from build123d import *

# Parameters (mm, degrees)
SKETCH1_W           = 12
SKETCH1_H           = 4.5
BOSS_EXTRUDE1_DEPTH = 12.23
BOSS_EXTRUDE2_DEPTH = 18.87
SKETCH3_R           = 3.225
BOSS_EXTRUDE3_DEPTH = 7.3
SKETCH4_R           = 1.6
BOSS_EXTRUDE4_DEPTH = 1


with BuildPart() as part:
    # Sketch1 → Boss-Extrude1 (new body)
    with BuildSketch(Plane(origin=(0, 0, 0), x_dir=(1, 0, 0), z_dir=(0, 1, 0))):
        Rectangle(SKETCH1_W, SKETCH1_H)
    extrude(amount=BOSS_EXTRUDE1_DEPTH)

    # Sketch2 → Boss-Extrude2 (add)
    with BuildSketch(Plane(origin=(0, 12.23, 0), x_dir=(1, 0, 0), z_dir=(0, 1, 0))):
        with BuildLine():
            Line((-6.025, -3.875), (6.025, -3.875))
            ThreePointArc((6.025, -3.875), (7.085660172, -3.435660172), (7.525, -2.375))
            Line((7.525, -2.375), (7.525, 2.375))
            ThreePointArc((7.525, 2.375), (7.085660172, 3.435660172), (6.025, 3.875))
            Line((6.025, 3.875), (-6.025, 3.875))
            ThreePointArc((-6.025, 3.875), (-7.085660172, 3.435660172), (-7.525, 2.375))
            Line((-7.525, 2.375), (-7.525, -2.375))
            ThreePointArc((-7.525, -2.375), (-7.085660172, -3.435660172), (-6.025, -3.875))
        make_face()
    extrude(amount=BOSS_EXTRUDE2_DEPTH)

    # Sketch3 → Boss-Extrude3 (add)
    with BuildSketch(Plane(origin=(0, 31.1, 0), x_dir=(1, 0, 0), z_dir=(0, 1, 0))):
        with Locations(Location((0, 0, 0), (0, 0, 90))):
            Circle(SKETCH3_R)
    extrude(amount=BOSS_EXTRUDE3_DEPTH)

    # Sketch4 → Boss-Extrude4 (add)
    with BuildSketch(Plane(origin=(0, 38.4, 0), x_dir=(1, 0, 0), z_dir=(0, 1, 0))):
        with Locations(Location((0, 0, 0), (0, 0, 270))):
            Circle(SKETCH4_R)
    extrude(amount=BOSS_EXTRUDE4_DEPTH)


solid = part.part
The model under review builds one solid part; all positions refer to its coordinate system, in mm. A direction names the side the tool comes from. Round coordinates to 2 decimals unless told otherwise and drop trailing zeros. Order: outer loops, then holes, each group sorted by start corner. A loop starts at its lowest first (then second) coordinate and runs counter-clockwise, first axis right, second up. Notation, with made-up numbers: (29.25, 8) - (62.25, 8) arc R20 cw to (62.25, 31) - close; hole circle Ø3 at (-39.75, 14). An arc over 180 degrees is marked (long way). Use one line per item in the form item = value.
Q1. Clearance check with flat-ended pins moving along their axes: P1, Ø3.5, axis at x = -2.5, y = 5, coming from the -Z side; P2, Ø1.5, axis at y = 5.5, z = 0, coming from the +X side; P3, Ø1.5, axis at x = -4, z = -0.5, coming from the +Y side. State where each tip first meets the part, or that it passes through.
Response values:
P1 = -2.25
P2 = 6
P3 = 31.1
Q2. Add section C-C on y = 27. Give the boundary of the cut face in (x, z) (3 decimals).
Response values:
outline = (-7.525, -2.375) arc R1.5 ccw to (-6.025, -3.875) - (6.025, -3.875) arc R1.5 ccw to (7.525, -2.375) - (7.525, 2.375) arc R1.5 ccw to (6.025, 3.875) - (-6.025, 3.875) arc R1.5 ccw to (-7.525, 2.375) - close
Q3. Add section D-D on x = -5.5. Give the boundary of the cut face in (y, z) (3 decimals).
Response values:
outline = (0, -2.25) - (12.23, -2.25) - (12.23, -3.875) - (31.1, -3.875) - (31.1, 3.875) - (12.23, 3.875) - (12.23, 2.25) - (0, 2.25) - close
Q4. To check wall thickness, follow line 1 (X direction, y = 4, z = 1.25); line 2 (Y direction, x = 4.25, z = -1); line 3 (Y direction, x = -0.5, z = 2.5). State the ranges of each line that lie inside material, in increasing order.
Response values:
line_1 = -6 to 6
line_2 = 0 to 31.1
line_3 = 12.23 to 38.4
Q5. Add section B-B on x = 0. Give the boundary of the cut face in (y, z) (3 decimals).
Response values:
outline = (0, -2.25) - (12.23, -2.25) - (12.23, -3.875) - (31.1, -3.875) - (31.1, -3.225) - (38.4, -3.225) - (38.4, -1.6) - (39.4, -1.6) - (39.4, 1.6) - (38.4, 1.6) - (38.4, 3.225) - (31.1, 3.225) - (31.1, 3.875) - (12.23, 3.875) - (12.23, 2.25) - (0, 2.25) - close
Q6. Tool access review of faces 1 (the cylindrical face through (3.15, 34.7, 0.7)), 2 (the flat face through (0, 6, -2.25)), 3 (the flat face through (0, 6, 2.25)): name each direction out of +Z, -Z, +X, -X, +Y, -Y from which nothing blocks a thin tool from reaching the whole face with its end or side.
Response values:
face_1 = +Y
face_2 = -Z, +X, -X, -Y
face_3 = +Z, +X, -X, -Y
Q7. Add section A-A on z = 0. Give the boundary of the cut face in (x, y) (3 decimals), then the cut area to 3 significant figures.
Response values:
outline = (-7.525, 12.23) - (-6, 12.23) - (-6, 0) - (6, 0) - (6, 12.23) - (7.525, 12.23) - (7.525, 31.1) - (3.225, 31.1) - (3.225, 38.4) - (1.6, 38.4) - (1.6, 39.4) - (-1.6, 39.4) - (-1.6, 38.4) - (-3.225, 38.4) - (-3.225, 31.1) - (-7.525, 31.1) - close
area = 481 mm^2
